Check sheet for the modelled part. Datum: model origin and axes. Units: mm. Round coordinates to 2 decimals unless told otherwise and drop trailing zeros. Write each loop counter-clockwise with the first axis right and the second up, starting at its lowest first coordinate (ties: lowest second). Pieces come first, ordered by that corner, then holes. Notation, with made-up numbers: M 14,47.5 L 54,47.5 A20 ccw 54,68.5 Z; hole C 24.25,-23.75 d2. An arc over 180 degrees is marked long. Put each result on its own line as item: value.
```python
from build123d import *

# Parameters (mm, degrees)
SKETCH1_R           = 30.5
BOSS_EXTRUDE1_DEPTH = 5
SKETCH4_R           = 3.302
CUT_EXTRUDE2_DEPTH  = 5.08
SKETCH5_R           = 3.302
CUT_EXTRUDE3_DEPTH  = 5.08
SKETCH6_R           = 3.302
CUT_EXTRUDE4_DEPTH  = 5.08


with BuildPart() as part:
    # Sketch1 → Boss-Extrude1 (new body)
    with BuildSketch(Plane(origin=(0, 0, 0), x_dir=(1, 0, 0), z_dir=(0, 1, 0))):
        with Locations(Location((0, 0, 0), (0, 0, 270))):
            Circle(SKETCH1_R)
    extrude(amount=BOSS_EXTRUDE1_DEPTH)

    # Sketch4 → Cut-Extrude2 (cut)
    with BuildSketch(Plane(origin=(0, 0, 0), x_dir=(-1, 0, 0), z_dir=(0, -1, 0))):
        with Locations(Location((0, 25, 0), (0, 0, 90))):
            Circle(SKETCH4_R)
    extrude(amount=-CUT_EXTRUDE2_DEPTH, mode=Mode.SUBTRACT)

    # Sketch5 → Cut-Extrude3 (cut)
    with BuildSketch(Plane.XZ):
        with Locations(Location((0, 25, 0), (0, 0, 270))):
            Circle(SKETCH5_R)
    extrude(amount=-CUT_EXTRUDE3_DEPTH, mode=Mode.SUBTRACT)

    # Sketch6 → Cut-Extrude4 (cut)
    with BuildSketch(Plane.XZ):
        with Locations(Location((17.674476483, 17.680862, 0), (0, 0, 270))):
            Circle(SKETCH6_R)
    extrude(amount=-CUT_EXTRUDE4_DEPTH, mode=Mode.SUBTRACT)


solid = part.part
```
1. Cross-section at A-A (x = 0). Enter the section's corners in (y, z), then the cut area to 3 significant figures.
Computed values:
outline: M 0,-30.5 L 5,-30.5 L 5,-28.3 L 0,-28.3 Z; M 0,-21.7 L 5,-21.7 L 5,21.7 L 0,21.7 Z; M 0,28.3 L 5,28.3 L 5,30.5 L 0,30.5 Z
area: 239 mm2
2. Cross-section at D-D (y = 3.25). Enter the section's corners in (x, z), then the cut area to 3 significant figures.
Computed values:
outline: C 0,0 d61; hole C 0,-25 d6.6; hole C 0,25 d6.6; hole C 17.67,17.68 d6.6
area: 2,820 mm2
3. Depth check by flat-ended pin: pin 1 Ø4 at (x, z) = (17.67, 17.68) entering from +Y; pin 2 Ø1.5 at (y, z) = (1, 1.5) entering from +X; pin 3 Ø1 at (x, y) = (-3, 4) entering from +Z; pin 4 Ø6 at (x, z) = (5.5, 22) entering from -Y. Enter the tip coordinate at first touch or a pass-through.
Computed values:
pin 1: passes through
pin 2: stops at x = 30.49
pin 3: stops at z = 30.4
pin 4: stops at y = 0
4. Release check for a two-part mould opening along X. For faces 1 (the cylindrical face through (0.99, 2.46, -28.15)), 2 (the flat face through (0, 0, 0)), 3 (the cylindrical face through (15.665, 2.465, 20.301)), 4 (the cylindrical face through (-29.775, 2.465, -6.612)) record: +X half, -X half, draft (parallel to the pull), parting line (faces both ways), or undercut.
Computed values:
face 1: undercut
face 2: draft
face 3: undercut
face 4: parting line
5. Cross-section at C-C (z = 23.5). Enter the section's corners in (x, y), then the cut area to 3 significant figures.
Computed values:
outline: M -19.44,0 L -2.94,0 L -2.94,5 L -19.44,5 Z; M 2.94,0 L 19.44,0 L 19.44,5 L 2.94,5 Z
area: 165 mm2
6. Cross-section at B-B (z = -24). Enter the section's corners in (x, y), then the cut area to 3 significant figures.
Computed values:
outline: M -18.82,0 L -3.15,0 L -3.15,5 L -18.82,5 Z; M 3.15,0 L 18.82,0 L 18.82,5 L 3.15,5 Z
area: 157 mm2
7. Scan lines: probe 1 along Z at (x, y) = (18, 2.95); probe 2 along X at (y, z) = (0.9, -0.5); probe 3 along X at (y, z) = (3.2, 25). Record each from-to range of solid material in increasing order.
Computed values:
probe 1: z = -24.62 to 14.39, 20.97 to 24.62
probe 2: x = -30.5 to 30.5
probe 3: x = -17.47 to -3.3, 3.3 to 17.47
